from build123d import *

# Parameters (mm, degrees)
F1_DEPTH = 25
F2_R     = 11
F3_R     = 3
F4_R     = 3
F6_D     = 10.5


with BuildPart() as f1:
    # F0 (on Top) → F1 (new body)
    with BuildSketch(Plane.XY):
        with BuildLine():
            ThreePointArc((-42.475013, 13.076226), (-42.211382, 17.110535), (-41.424972, 21.076226))
            Line((-41.424972, 21.076226), (-66.424972, 21.076226))
            Line((-66.424972, 21.076226), (-66.424972, 13.076226))
            Line((-66.424972, 13.076226), (-42.475013, 13.076226))
        make_face()
        with BuildLine():
            Line((43.474945, 21.076226), (18.474945, 21.076226))
            ThreePointArc((18.474945, 21.076226), (19.261355, 17.110535), (19.524987, 13.076226))
            Line((19.524987, 13.076226), (43.474945, 13.076226))
            Line((43.474945, 13.076226), (43.474945, 21.076226))
        make_face()
        with BuildLine():
            ThreePointArc((18.474945, 21.076226), (7.406194, 37.662808), (-11.475013, 44.076226))
            ThreePointArc((-11.475013, 44.076226), (-30.356221, 37.662808), (-41.424972, 21.076226))
            ThreePointArc((-41.424972, 21.076226), (-42.211382, 17.110535), (-42.475013, 13.076226))
            Line((-42.475013, 13.076226), (-35.475013, 13.076226))
            ThreePointArc((-35.475013, 13.076226), (-28.445576, 30.046789), (-11.475013, 37.076226))
            ThreePointArc((-11.475013, 37.076226), (5.495549, 30.046789), (12.524987, 13.076226))
            Line((12.524987, 13.076226), (19.524987, 13.076226))
            ThreePointArc((19.524987, 13.076226), (19.261355, 17.110535), (18.474945, 21.076226))
        make_face()
    extrude(amount=F1_DEPTH)

    # F2
    f2_edges = [f1.edges().sort_by_distance(p)[0] for p in [
        (43.474945, 17.076226, 0),
        (43.474945, 17.076226, 25),
        (-66.424972, 17.076226, 25),
        (-66.424972, 17.076226, 0),
    ]]
    fillet(f2_edges, radius=F2_R)

    # F3
    f3_edges = [f1.edges().sort_by_distance(p)[0] for p in [
        (-35.475013, 13.076226, 12.5),
        (12.524987, 13.076226, 12.5),
    ]]
    fillet(f3_edges, radius=F3_R)

    # F4
    f4_edges = [f1.edges().sort_by_distance(p)[0] for p in [
        (-41.424972, 21.076226, 12.5),
        (18.474945, 21.076226, 12.5),
    ]]
    fillet(f4_edges, radius=F4_R)

    # F6 (through all)
    with Locations(Plane(origin=(0, 21.076226, 0), x_dir=(-1, 0, 0), z_dir=(0, 1, 0))):
        with Locations((55.174972, 12.5), (-32.224945, 12.5)):
            Hole(F6_D / 2)


solid = f1.part
Read the model definition and answer for the solid it produces. Units are mm, in the model's axes. A direction names the side the tool comes from. Give positions to 0.01 mm unless a question says otherwise; leave off trailing zeros. Loops run counter-clockwise (first coordinate to the right, second up) from the corner with the lowest first, then second, coordinate; pieces in that order, holes last. Notation, with made-up numbers: (67, 51) -> (112, 51) arc R21 cw to (112, 79) -> close; hole circle Ø6 at (34.5, 79). An arc over 180 degrees is marked (long way). Answer as CSV lines item,"result".
Item 1: Each of these flat-tipped pins is pushed along its axis until it touches: pin 1 (11.5 mm diameter, centred on x = -54.5, z = 11, fed in from +Y); pin 2 (8 mm diameter, centred on y = 38.5, z = 9, fed in from +X); pin 3 (2 mm diameter, centred on x = -29, z = 8.5, fed in from -Y); pin 4 (9.5 mm diameter, centred on x = 32.22, z = 12.5, fed in from +Y). Where does it stop, or does it pass through?
Returned:
pin 1,"stops at y = 21.08"
pin 2,"stops at x = 10.93"
pin 3,"stops at y = 28.33"
pin 4,"passes through"
Item 2: Find section A-A on z = 12.5. Give the vertices of the cut face in (x, y), plus the area to 3 significant figures.
Returned:
outline,"(-66.42, 13.08) -> (-60.42, 13.08) -> (-60.42, 21.08) -> (-66.42, 21.08) -> close; (-49.92, 13.08) -> (-38.31, 13.08) arc R3 ccw to (-35.33, 15.74) arc R24 cw to (-11.48, 37.08) arc R24 cw to (12.38, 15.74) arc R3 ccw to (15.36, 13.08) -> (26.97, 13.08) -> (26.97, 21.08) -> (20.7, 21.08) arc R3 cw to (17.86, 23.11) arc R31 ccw to (-40.81, 23.11) arc R3 cw to (-43.65, 21.08) -> (-49.92, 21.08) -> close; (37.47, 13.08) -> (43.47, 13.08) -> (43.47, 21.08) -> (37.47, 21.08) -> close"
area,"824 mm²"
Item 3: Find section C-C on z = 3.5. Give the vertices of the cut face in (x, y), plus the area to 3 significant figures.
Returned:
outline,"(-63.47, 13.08) -> (-38.31, 13.08) arc R3 ccw to (-35.33, 15.74) arc R24 cw to (-11.48, 37.08) arc R24 cw to (12.38, 15.74) arc R3 ccw to (15.36, 13.08) -> (40.52, 13.08) -> (40.52, 21.08) -> (20.7, 21.08) arc R3 cw to (17.86, 23.11) arc R31 ccw to (-40.81, 23.11) arc R3 cw to (-43.65, 21.08) -> (-63.47, 21.08) -> close"
area,"945 mm²"
Item 4: Find section D-D on y = 33.5. Give the vertices of the cut face in (x, z), plus the area to 3 significant figures.
Returned:
outline,"(-34.8, 0) -> (-24.08, 0) -> (-24.08, 25) -> (-34.8, 25) -> close; (1.13, 0) -> (11.85, 0) -> (11.85, 25) -> (1.13, 25) -> close"
area,"536 mm²"
Item 5: Consider line 1 (X direction, y = 16, z = 11); line 2 (Y direction, x = -44.5, z = 14); line 3 (X direction, y = 21, z = 4.75). Determine where each line is inside the solid, lowest interval first. Write a range as [from, to].
Returned:
line 1,"x = [-66.42, -60.21], [-50.14, -35.3], [12.35, 27.19], [37.26, 43.47]"
line 2,"y = [13.08, 21.08]"
line 3,"x = [-64.48, -34.13], [11.18, 41.53]"
Item 6: For faces 1 (the face through (27, 21.076, 10)), 2 (the face through (43.475, 17, 12)), 3 (the face through (40.34, 17.13, 21.69)), 4 (the face through (13.335, 13.861, 12.675)), 5 (the face through (-50, 21.076, 10)), determine the directions among +Z, -Z, +X, -X, +Y, -Y from which every point of the face is accessible in a straight line to the end or side of a thin tool.
Returned:
face 1,"+Z, -Z, +X, +Y"
face 2,"+Z, -Z, +X, +Y, -Y"
face 3,"+Z, +X, +Y, -Y"
face 4,"+Z, -Z, -Y"
face 5,"+Z, -Z, -X, +Y"
Item 7: Find section B-B on y = 27.5. Give the vertices of the cut face in (x, z) (3 decimals).
Returned:
outline,"(-38.915, 0) -> (-30.657, 0) -> (-30.657, 25) -> (-38.915, 25) -> close; (7.707, 0) -> (15.965, 0) -> (15.965, 25) -> (7.707, 25) -> close"
Item 8: Determine the mould class of faces 6 (the face through (28.355, 17.02, 16.048)), 7 (the face through (18.93, 21.65, 12.68)), 8 (the face through (-63.29, 17.02, 21.69)), 9 (the face through (-50.17, 17.02, 14.08)) for opening direction Z: +Z half, -Z half, draft (parallel to the pull), parting line (faces both ways), or undercut.
Returned:
face 6,"undercut"
face 7,"draft"
face 8,"+Z half"
face 9,"undercut"
